Can you work these out from the model? Positions are in its coordinate system, mm. Round coordinates to 2 decimals unless told otherwise and drop trailing zeros. Loops run counter-clockwise (first coordinate to the right, second up) from the corner with the lowest first, then second, coordinate; pieces in that order, holes last.
```python
from build123d import *

# Parameters (mm, degrees)
SKETCH1_W           = 36
SKETCH1_H           = 36
SKETCH1_R           = 1.5
BOSS_EXTRUDE1_DEPTH = 1.6
FILLET1_R           = 2
CUT_EXTRUDE1_DEPTH  = 0.01


with BuildPart() as part:
    # Sketch1 → Boss-Extrude1 (new body)
    with BuildSketch(Plane(origin=(0, 0, 0), x_dir=(1, 0, 0), z_dir=(0, 1, 0))):
        Rectangle(SKETCH1_W, SKETCH1_H)
        with Locations(Location((-15.5, 15.5, 0), (0, 0, 270))):
            Circle(SKETCH1_R, mode=Mode.SUBTRACT)
        with Locations(Location((15.5, 15.5, 0), (0, 0, 270))):
            Circle(SKETCH1_R, mode=Mode.SUBTRACT)
        with Locations(Location((-15.5, -15.5, 0), (0, 0, 90))):
            Circle(SKETCH1_R, mode=Mode.SUBTRACT)
        with Locations(Location((15.5, -15.5, 0), (0, 0, 90))):
            Circle(SKETCH1_R, mode=Mode.SUBTRACT)
    extrude(amount=BOSS_EXTRUDE1_DEPTH)

    # Fillet1
    fillet1_edges = [part.edges().sort_by_distance(p)[0] for p in [
        (18, 0.8, 18),
        (-18, 0.8, 18),
        (-18, 0.8, -18),
        (18, 0.8, -18),
    ]]
    fillet(fillet1_edges, radius=FILLET1_R)

    # Sketch2 → Cut-Extrude1 (cut)
    with BuildSketch(Plane(origin=(0, 1.6, 0), x_dir=(1, 0, 0), z_dir=(0, 1, 0))):
        Polygon((-2.822286409, 1.851413804), (-1.117158204, 1.851413804), (-1.117158204, 1.492439445), (-2.508183845, 1.492439445), (-2.508183845, 0.415516368), (-1.117158204, 0.415516368), (-1.117158204, 0.056542009), (-2.508183845, 0.056542009), (-2.508183845, -1.648586196), (-2.822286409, -1.648586196), align=None)
        with BuildLine():
            Line((2.741816155, 1.209186239), (2.466976411, 0.998849701))
            add(Edge.make_bspline(
                [(2.466976411, 0.998849701), (2.447370523, 1.022215671), (2.408423076, 1.068632587), (2.345763874, 1.133812131), (2.280462231, 1.194877392), (2.212543109, 1.252119272), (2.14078399, 1.303536038), (2.066923191, 1.351807141), (1.989725146, 1.395074879), (1.882973411, 1.447537865), (1.743325563, 1.50228402), (1.567530724, 1.548187251), (1.384019626, 1.577408427), (1.258822026, 1.580573268), (1.195141475, 1.582183034)],
                knots=[0, 0, 0, 0, 0.757959112, 1.505699292, 2.245454638, 2.979532153, 3.711538275, 4.438200793, 5.171680507, 5.909471876, 7.393775596, 8.890124382, 10.418191784, 12, 12, 12, 12], degree=3))
            add(Edge.make_bspline(
                [(1.195141475, 1.582183034), (1.160058176, 1.581779072), (1.090217183, 1.580974896), (0.98656871, 1.570365771), (0.884855659, 1.555454561), (0.785144193, 1.533329238), (0.687561234, 1.505356618), (0.591468832, 1.471931205), (0.498258232, 1.430576365), (0.406639994, 1.384868105), (0.318860783, 1.33324066), (0.235805735, 1.276927308), (0.157777767, 1.216558212), (0.084715155, 1.151907105), (0.016543207, 1.083265145), (-0.046244104, 1.009900803), (-0.103429514, 0.93204863), (-0.156146539, 0.850735222), (-0.203359273, 0.76619743), (-0.242889152, 0.67812236), (-0.277894274, 0.588018257), (-0.305593517, 0.494867096), (-0.327518034, 0.39932433), (-0.342645697, 0.301133542), (-0.353134168, 0.200499863), (-0.353934345, 0.13229055), (-0.354337691, 0.097908195)],
                knots=[0, 0, 0, 0, 1.054917814, 2.100044995, 3.131103042, 4.146048494, 5.169673617, 6.183595914, 7.203665975, 8.234915748, 9.262203917, 10.264457458, 11.251630812, 12.227803204, 13.197192746, 14.159520551, 15.12972552, 16.100847026, 17.073214652, 18.039054194, 19.002613845, 19.979014051, 20.95965708, 21.949030935, 22.966165397, 24, 24, 24, 24], degree=3))
            add(Edge.make_bspline(
                [(-0.354337691, 0.097908195), (-0.353075872, 0.046176875), (-0.350598458, -0.05539071), (-0.328550124, -0.204161321), (-0.295045033, -0.346681994), (-0.244829456, -0.482061837), (-0.182910405, -0.611970195), (-0.104669794, -0.734209048), (-0.014053256, -0.850625613), (0.090221163, -0.958468561), (0.204626979, -1.056982286), (0.327374891, -1.143732867), (0.458159179, -1.21604775), (0.595535809, -1.276223696), (0.740561923, -1.322480424), (0.892976725, -1.355044547), (1.05244872, -1.376286728), (1.16141812, -1.378320416), (1.216876251, -1.379355427)],
                knots=[0, 0, 0, 0, 1.029171465, 2.020641659, 2.987623507, 3.938342917, 4.889210282, 5.84687017, 6.821220943, 7.821438502, 8.827599549, 9.822697543, 10.807740252, 11.797342354, 12.80366471, 13.83203677, 14.896651826, 16, 16, 16, 16], degree=3))
            add(Edge.make_bspline(
                [(1.216876251, -1.379355427), (1.27797894, -1.377666647), (1.398243649, -1.374342725), (1.574611675, -1.346183476), (1.743447441, -1.300525558), (1.904760027, -1.236627636), (2.058094674, -1.153562348), (2.203691334, -1.05286447), (2.341672904, -0.933576138), (2.424644187, -0.842493009), (2.466976411, -0.796022094)],
                knots=[0, 0, 0, 0, 1.028121516, 2.023589091, 2.998037872, 3.967518031, 4.937445131, 5.927275754, 6.942489185, 8, 8, 8, 8], degree=3))
            Line((2.466976411, -0.796022094), (2.741816155, -1.004255267))
            add(Edge.make_bspline(
                [(2.741816155, -1.004255267), (2.719698045, -1.032793719), (2.67556777, -1.089733925), (2.604109753, -1.170005635), (2.528832455, -1.24550967), (2.449176745, -1.315637292), (2.366058954, -1.381791757), (2.277986641, -1.442093588), (2.186117609, -1.497384473), (2.09076313, -1.548011397), (1.992024517, -1.592928644), (1.890020082, -1.631382412), (1.785189507, -1.664507302), (1.677527998, -1.691759238), (1.566812241, -1.713030322), (1.453441767, -1.727249997), (1.337171892, -1.736991911), (1.258730471, -1.737879827), (1.218979616, -1.738329786)],
                knots=[0, 0, 0, 0, 0.986787822, 1.968848986, 2.935600012, 3.899624008, 4.868462664, 5.837806735, 6.815139263, 7.798259679, 8.787526145, 9.778297419, 10.776456485, 11.791383307, 12.812564526, 13.85620153, 14.913611965, 16, 16, 16, 16], degree=3))
            add(Edge.make_bspline(
                [(1.218979616, -1.738329786), (1.181335949, -1.738067794), (1.106900259, -1.737549736), (0.997001508, -1.729157568), (0.890011927, -1.717707831), (0.786237301, -1.7004677), (0.685111326, -1.68012336), (0.587550741, -1.652852104), (0.492595531, -1.622302937), (0.40062719, -1.58639795), (0.311567491, -1.545881768), (0.225703679, -1.500090209), (0.143075247, -1.449408344), (0.062869826, -1.394953334), (-0.013727758, -1.334976032), (-0.087381283, -1.270309397), (-0.158503759, -1.201171387), (-0.202506444, -1.151316533), (-0.224630159, -1.126250459)],
                knots=[0, 0, 0, 0, 1.114604814, 2.203992996, 3.262667896, 4.300477797, 5.318619304, 6.316056647, 7.298880507, 8.271930387, 9.238335007, 10.195173496, 11.151986948, 12.108099108, 13.064862484, 14.031167946, 15.010108607, 16, 16, 16, 16], degree=3))
            add(Edge.make_bspline(
                [(-0.224630159, -1.126250459), (-0.260065803, -1.08270927), (-0.33050928, -0.99615256), (-0.420634963, -0.855866579), (-0.497782518, -0.70939837), (-0.560158439, -0.555978441), (-0.608921172, -0.395951054), (-0.642702367, -0.229235539), (-0.664653972, -0.055987597), (-0.667164261, 0.061849192), (-0.668440255, 0.121746336)],
                knots=[0, 0, 0, 0, 0.994628077, 1.977248131, 2.950237994, 3.925870899, 4.908910175, 5.911660606, 6.938484602, 8, 8, 8, 8], degree=3))
            add(Edge.make_bspline(
                [(-0.668440255, 0.121746336), (-0.666885062, 0.184701789), (-0.663825316, 0.308562714), (-0.63782952, 0.490336667), (-0.596010724, 0.664488066), (-0.536613835, 0.83069181), (-0.461308484, 0.989822091), (-0.36828187, 1.140663296), (-0.258614728, 1.284180095), (-0.13316716, 1.418194847), (0.004400175, 1.540734199), (0.151718989, 1.648540403), (0.308500936, 1.738257919), (0.473018788, 1.813254081), (0.646504469, 1.870898544), (0.828587838, 1.911251731), (1.018926753, 1.936368847), (1.148789179, 1.939544055), (1.214772886, 1.941157393)],
                knots=[0, 0, 0, 0, 1.032925535, 2.032216505, 3.007276963, 3.968222605, 4.92396291, 5.891752235, 6.871517503, 7.883894988, 8.900124299, 9.891468569, 10.874487609, 11.85992873, 12.854644235, 13.869047385, 14.917252991, 16, 16, 16, 16], degree=3))
            add(Edge.make_bspline(
                [(1.214772886, 1.941157393), (1.254987358, 1.940675255), (1.334587855, 1.939720911), (1.452340507, 1.930414769), (1.566982834, 1.914901163), (1.678593816, 1.893785093), (1.787716432, 1.867577772), (1.893516673, 1.833437473), (1.99661536, 1.794400942), (2.096362268, 1.749442476), (2.192278819, 1.698975735), (2.284335137, 1.643560111), (2.371799996, 1.583264305), (2.455288844, 1.51860113), (2.533405055, 1.448202571), (2.608366534, 1.374004975), (2.677627612, 1.293871151), (2.720380807, 1.237466217), (2.741816155, 1.209186239)],
                knots=[0, 0, 0, 0, 1.096760587, 2.17092713, 3.219439832, 4.250915756, 5.268269357, 6.278326846, 7.281116186, 8.274029601, 9.260640565, 10.235837813, 11.203064059, 12.156899882, 13.114053108, 14.069676657, 15.032185724, 16, 16, 16, 16], degree=3))
        make_face()
    extrude(amount=-CUT_EXTRUDE1_DEPTH, mode=Mode.SUBTRACT)


solid = part.part
```
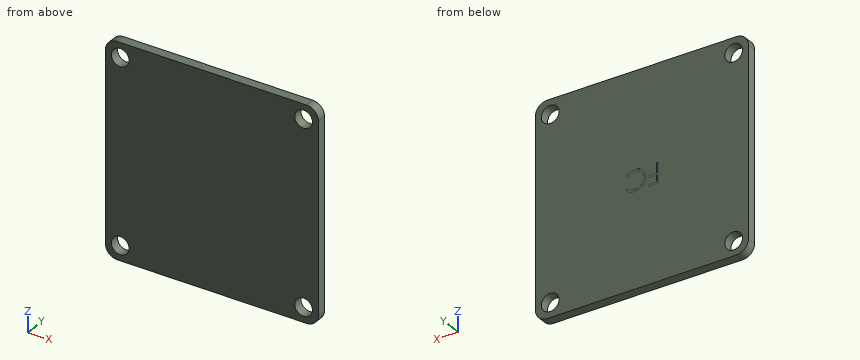
(1) If I drill on line 1 (X direction, y = 0.6, z = -15.5); line 2 (Y direction, x = -0.5, z = 0), over which ranges is the centre line in solid material (lowest first)?
(2) Suppose I cut it at C-C (y = 1.05). Write out the boundary of the cut face in (x, z), then the cut area to 3 significant figures.
(3) Suppose I cut it at A-A (z = 15.5). Write out the boundary of the cut face in (x, y).
(4) Suppose I cut it at B-B (x = -15.5). Write out the boundary of the cut face in (y, z).
Check result:
1. line 1: x = -18 to -17, -14 to 14, 17 to 18
1. line 2: y = 0 to 1.59
2. outline: (-18, -16) arc R2 ccw to (-16, -18) - (16, -18) arc R2 ccw to (18, -16) - (18, 16) arc R2 ccw to (16, 18) - (-16, 18) arc R2 ccw to (-18, 16) - close; hole circle Ø3 at (-15.5, -15.5); hole circle Ø3 at (-15.5, 15.5); hole circle Ø3 at (15.5, -15.5); hole circle Ø3 at (15.5, 15.5)
2. area: 1,260 mm2
3. outline: (-18, 0) - (-17, 0) - (-17, 1.6) - (-18, 1.6) - close; (-14, 0) - (14, 0) - (14, 1.6) - (-14, 1.6) - close; (17, 0) - (18, 0) - (18, 1.6) - (17, 1.6) - close
4. outline: (0, -18) - (1.6, -18) - (1.6, -17) - (0, -17) - close; (0, -14) - (1.6, -14) - (1.6, 14) - (0, 14) - close; (0, 17) - (1.6, 17) - (1.6, 18) - (0, 18) - close
